```python
from build123d import *

# Parameters (mm, degrees)
SKETCH_1_W           = 37
SKETCH_1_H           = 18
EXTRUDE_1_DEPTH      = 10
EXTRUDE_2_DEPTH      = 8
EXTRUDE_2_DEPTH_BACK = 45
SKETCH_2_W           = 9
SKETCH_2_H           = 2
SKETCH_3_R           = 1.75
CUT_EXTRUDE_1_DEPTH  = 8


with BuildPart() as part:
    # 草图1 → 凸台-拉伸1 (new body)
    with BuildSketch(Plane(origin=(0, 0, 0), x_dir=(1, 0, 0), z_dir=(0, 1, 0))):
        with Locations((-27.266289308, 19.375099371)):
            Rectangle(SKETCH_1_W, SKETCH_1_H)
    extrude(amount=EXTRUDE_1_DEPTH)

    # 草图2 → 凸台-拉伸2 (add, two sides: drawn at the far end of the back side and taken through both)
    with BuildSketch(Plane.ZY.offset(45.766289308).offset(-EXTRUDE_2_DEPTH_BACK)):
        with Locations((-19.375099371, 4)):
            Rectangle(SKETCH_2_W, SKETCH_2_H)
    extrude(amount=EXTRUDE_2_DEPTH + EXTRUDE_2_DEPTH_BACK)

    # 草图3 → 切除-拉伸1 (cut)
    with BuildSketch(Plane(origin=(0, 5, 0), x_dir=(1, 0, 0), z_dir=(0, 1, 0))):
        with Locations(Location((-49.766289308, 19.375099371, 0), (0, 0, 270))):
            Circle(SKETCH_3_R)
        with Locations(Location((-4.766289308, 19.375099371, 0), (0, 0, 270))):
            Circle(SKETCH_3_R)
    extrude(amount=-CUT_EXTRUDE_1_DEPTH, mode=Mode.SUBTRACT)


solid = part.part
```
CAD build for the part. Positions are in the model's coordinates, mm. A direction names the side the tool comes from. Coordinates: 2 decimals unless noted, no trailing zeros. Order: outer loops, then holes, each group sorted by start corner. A loop starts at its lowest first (then second) coordinate and runs counter-clockwise, first axis right, second up. Notation, with made-up numbers: (13.25, 51) - (27.25, 51) arc R37 cw to (27.25, 90) - close; hole circle Ø10 at (-22, 28.25). An arc over 180 degrees is marked (long way). Answer in a Markdown table with one row per item.
1. Pull direction Z, two halves, no side cores. Call faces 6 (the face through (-0.766, 4, -19)), 7 (the face through (-51.475, 4.014, -19.754)), 8 (the face through (-50, 4, -14.875)), 9 (the face through (-6.475, 4.014, -19.754)): +Z half, -Z half, draft (parallel to the pull), parting line (faces both ways), or undercut.
Answer:
| item | result |
|---|---|
| face 6 | draft |
| face 7 | undercut |
| face 8 | +Z half |
| face 9 | undercut |
2. Drill centre lines: L1, parallel to X at y = 9, z = -11; L2, parallel to X at y = 3.25, z = -20.25; L3, parallel to Y at x = -50.5, z = -22. Where is each one in solid material? Low to high. Write a range as from..to.
Answer:
| item | result |
|---|---|
| L1 | -45.77..-8.77 |
| L2 | -53.77..-51.28, -48.25..-6.28, -3.25..-0.77 |
| L3 | 3..5 |
3. Flat gauge pins, fed straight in: P1, Ø3, axis at y = 6, z = -13, coming from the -X side; P2, Ø1.6, axis at x = -3, y = 4, coming from the +Z side; P3, Ø2.5, axis at x = -49.5, z = -17.5, coming from the +Y side; P4, Ø3, axis at x = -4.77, z = -19.38, coming from the -Y side. Where does each tip first touch, or does it go through?
Answer:
| item | result |
|---|---|
| P1 | x = -45.77 |
| P2 | z = -14.88 |
| P3 | y = 5 |
| P4 | through |
4. Slice it at A-A, the plane y = 3.75. List the corners of the cut face in (x, z).
Answer:
| item | result |
|---|---|
| outline | (-53.77, -23.88) - (-45.77, -23.88) - (-45.77, -28.38) - (-8.77, -28.38) - (-8.77, -23.88) - (-0.77, -23.88) - (-0.77, -14.88) - (-8.77, -14.88) - (-8.77, -10.38) - (-45.77, -10.38) - (-45.77, -14.88) - (-53.77, -14.88) - close; hole circle Ø3.5 at (-49.77, -19.38); hole circle Ø3.5 at (-4.77, -19.38) |
5. 3-axis set-ups, long thin cutter, end or side, ignore diameter. For faces 1 (the face through (-5, 5, -17)), 2 (the face through (-50, 5, -17)), 3 (the face through (-5, 3, -17)), 4 (the face through (-5, 4, -23.875)), 5 (the face through (-50, 4, -23.875)): which of +Z, -Z, +X, -X, +Y, -Y reach the whole face in a straight line?
Answer:
| item | result |
|---|---|
| face 1 | +Z, -Z, +X, +Y |
| face 2 | +Z, -Z, -X, +Y |
| face 3 | +Z, -Z, +X, -Y |
| face 4 | -Z, +X, +Y, -Y |
| face 5 | -Z, -X, +Y, -Y |
6. Slice it at D-D, the plane z = -20. List the corners of the cut face in (x, y), then the cut area to 3 significant figures.
Answer:
| item | result |
|---|---|
| outline | (-53.77, 3) - (-51.4, 3) - (-51.4, 5) - (-53.77, 5) - close; (-48.13, 3) - (-45.77, 3) - (-45.77, 0) - (-8.77, 0) - (-8.77, 3) - (-6.4, 3) - (-6.4, 5) - (-8.77, 5) - (-8.77, 10) - (-45.77, 10) - (-45.77, 5) - (-48.13, 5) - close; (-3.13, 3) - (-0.77, 3) - (-0.77, 5) - (-3.13, 5) - close |
| area | 389 mm² |
7. Slice it at C-C, the plane z = -16. List the corners of the cut face in (x, y), then the cut area to 3 significant figures.
Answer:
| item | result |
|---|---|
| outline | (-53.77, 3) - (-45.77, 3) - (-45.77, 0) - (-8.77, 0) - (-8.77, 3) - (-0.77, 3) - (-0.77, 5) - (-8.77, 5) - (-8.77, 10) - (-45.77, 10) - (-45.77, 5) - (-53.77, 5) - close |
| area | 402 mm² |
8. Slice it at B-B, the plane x = -49. List the corners of the cut face in (y, z).
Answer:
| item | result |
|---|---|
| outline | (3, -23.88) - (5, -23.88) - (5, -20.95) - (3, -20.95) - close; (3, -17.8) - (5, -17.8) - (5, -14.88) - (3, -14.88) - close |
